Verification items for the finished model (mm, model axes). A direction names the side the tool comes from. Coordinates: 2 decimals unless noted, no trailing zeros. Order: outer loops, then holes, each group sorted by start corner. A loop starts at its lowest first (then second) coordinate and runs counter-clockwise, first axis right, second up.
Q1. Cross-section at C-C, the plane z = 18. Record the boundary of the cut face in (x, y).
Q2. Cross-section at B-B, the plane x = 7. Record the boundary of the cut face in (y, z), and give its area (3 significant figures).
Q3. Draft check along Y on faces 1 (the conical face through (12.33, -7.43, 15.14)), 2 (the conical face through (0.1, -14.4, 15.3)), 3 (the cylindrical face through (-17.56, -10.226, 13.274)), 4 (the cylindrical face through (-5.47, -24.65, 14.93)). Enter one of: pulls with the +Y half, pulls with the -Y half, needs draft (parallel to the pull), parting line crosses it, or undercut.
Q4. Cross-section at A-A, the plane z = 7. Record the boundary of the cut face in (x, y), and give its area (3 significant figures).
Q5. Depth check by flat-ended pin: P1, Ø5, axis at y = 11.5, z = 9.5, coming from the +X side; P2, Ø12, axis at y = -12, z = 8.5, coming from the +X side; P3, Ø2.5, axis at x = 0.5, y = 0.5, coming from the +Z side. Enter the tip coordinate at first touch or a pass-through.
Q6. Thickness scan on line 1 (Y direction, x = -15, z = 14); line 2 (Z direction, x = 14, y = -8); line 3 (Y direction, x = 0, z = 9). Record the ranges inside material, lowest first.
Q7. Set-up check for faces 5 (the cylindrical face through (0.076, -20.32, 13.274)), 6 (the cylindrical face through (2.988, -22.755, 8.175)), 7 (the conical face through (0.715, 0.159, 2.907)), 8 (the cylindrical face through (-0.076, 20.32, 13.274)): record each of +Z, -Z, +X, -X, +Y, -Y from which the full face is reachable in a straight line by a thin tool's end or side.
from build123d import *

# Parameters (mm, degrees)
SKETCH2_R           = 25.25
BOSS_EXTRUDE1_DEPTH = 20
SKETCH3_W           = 3.6
SKETCH3_H           = 2.3
CIRPATTERN1_COUNT   = 6


with BuildPart() as part:
    # Sketch2 → Boss-Extrude1 (new body)
    with BuildSketch(Plane.XY):
        Circle(SKETCH2_R)
    extrude(amount=BOSS_EXTRUDE1_DEPTH)

    # Sketch3 → Cut-Revolve1 (revolve, cut)
    with BuildSketch(Plane(origin=(0, 0, 0), x_dir=(0, 0, -1), z_dir=(1, 0, 0)), mode=Mode.PRIVATE) as cut_revolve1_sk:
        with Locations((-8.2, 24.1)):
            Rectangle(SKETCH3_W, SKETCH3_H)
    revolve(cut_revolve1_sk.sketch.rotate(Axis((0, 0, 0), (0, 0, 1)), 90), axis=Axis((0, 0, 0), (0, 0, 1)), mode=Mode.SUBTRACT)

    # Sketch7 → #8-32 Tapped Hole2 (revolve, cut)
    with BuildSketch(Plane(origin=(0, 25.25, 15), x_dir=(0, 0, 1), z_dir=(1, 0, 0))):
        Polygon((0, 0), (0, 11.037806461), (1.7272, 10), (1.7272, 0), align=None)
    f_8_32_tapped_hole2 = revolve(axis=Axis((0, 31.6, 15), (0, -1, 0)), mode=Mode.SUBTRACT)

    # CirPattern1: #8-32 Tapped Hole2 ×6 about axis
    cirpattern1_axis = Axis((0, 0, 21.768762267), (0, 0, -1))
    for i in range(1, CIRPATTERN1_COUNT):
        add(f_8_32_tapped_hole2.rotate(cirpattern1_axis, i * 360 / CIRPATTERN1_COUNT), mode=Mode.SUBTRACT)

    # Sketch11 → 1/8 NPT Tapped Hole1 (revolve, cut)
    with BuildSketch(Plane(origin=(0, 0, 20), x_dir=(0, -1, 0), z_dir=(1, 0, 0))):
        Polygon((0, 0), (0, 17.533468714), (4.2164, 15), (4.2164, 6.92), (4.528555848, 6.92), (4.744593, 0), align=None)
    revolve(axis=Axis((0, 0, 26.35), (0, 0, -1)), mode=Mode.SUBTRACT)


solid = part.part
Check values:
1. outline: circle Ø50.5 at (0, 0); hole circle Ø9.36 at (0, 0)
2. outline: (-24.26, 0) - (24.26, 0) - (24.26, 6.4) - (21.86, 6.4) - (21.86, 10) - (24.26, 10) - (24.26, 20) - (-24.26, 20) - (-24.26, 10) - (-21.86, 10) - (-21.86, 6.4) - (-24.26, 6.4) - close
2. area: 953 mm2
3. face 1: undercut
3. face 2: pulls with the -Y half
3. face 3: undercut
3. face 4: parting line crosses it
4. outline: circle Ø45.9 at (0, 0); hole circle Ø8.43 at (0, 0)
4. area: 1,600 mm2
5. P1: stops at x = 23.57
5. P2: stops at x = 24.48
5. P3: stops at z = 3.64
6. line 1: y = -20.31 to -10.29, -7.03 to 7.03, 10.29 to 20.31
6. line 2: z = 0 to 13.27, 16.73 to 20
6. line 3: y = -22.95 to -4.22, 4.22 to 22.95
7. face 5: -Y
7. face 6: none
7. face 7: +Z
7. face 8: +Y
